Can you work these out from the model? Positions are in its coordinate system, mm. Face numbers are marked on the shaded views. A direction names the side the tool comes from. Round coordinates to 2 decimals unless told otherwise and drop trailing zeros. Order: outer loops, then holes, each group sorted by start corner. A loop starts at its lowest first (then second) coordinate and runs counter-clockwise, first axis right, second up. Notation, with made-up numbers: (89, -18) -> (111, -18) arc R15 cw to (111, 7) -> close; hole circle Ø11 at (20, 15.5). An arc over 180 degrees is marked (long way). Use a Markdown table: item, result. Add a question column.
Q1. We'd pull the mould along X, two halves only. Please class the marked faces 3, 4 and 5: +X half, -X half, draft (parallel to the pull), parting line (faces both ways), or undercut.
Q2. I'm going to push flat-ended pins straight in: pin 1 Ø11.5 at (x, y) = (0, 0) entering from +Z; pin 2 Ø1.5 at (y, z) = (-82.5, -3.5) entering from +X; pin 3 Ø17 at (x, y) = (0, 0) entering from +Z. Where does each tip first touch, or does it pass through?
Q3. For the marked faces 1 and 2, which set-ups out of +Z, -Z, +X, -X, +Y, -Y let a thin tool reach every point of the face, with its end or its side?
Q4. If we section it at A-A on z = 0: List the corners of the cut face in (x, y) for me (3 decimals), plus the area to 3 significant figures.
Q5. I need wall thicknesses on line 1 along Y through (x, z) = (0, -25.5); line 2 along Z through (x, y) = (0, -65.5) (3 decimals); line 3 along Y through (x, z) = (25, 47). Which ranges of each line are inside material? Lowest first, please. Write a range as [from, to].
Q6. If we section it at B-B on y = 71: List the corners of the cut face in (x, z) for me (3 decimals), plus the area to 3 significant figures.
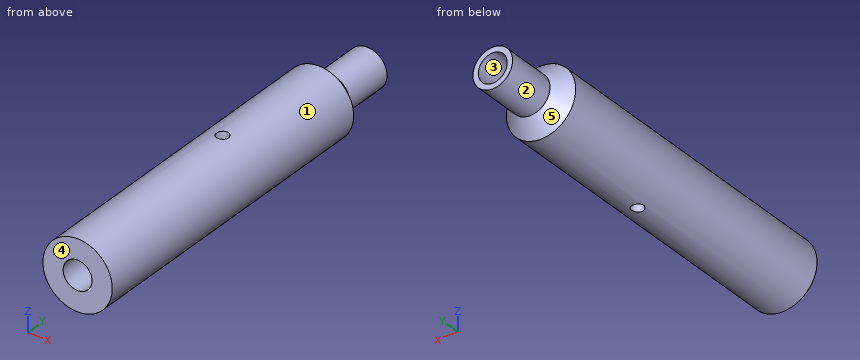
```python
from build123d import *

# Parameters (mm, degrees)
F0_R      = 53.34
F0_R_2    = 22.225
F1_DEPTH  = 304.8
F4_R      = 53.34
F4_R_2    = 30.48
F5_DEPTH  = 101.6
F10_R     = 9.525
F10_R_2   = 3.302
F11_DEPTH = 19.05
F12_DEPTH = 32.3616602869
F13_R     = 9.525
F13_R_2   = 3.302
F14_DEPTH = 19.05
F15_DEPTH = 32.3616602869


with BuildPart() as f1:
    # F0 (on Front) → F1 (new body, symmetric)
    with BuildSketch(Plane.XZ):
        Circle(F0_R)
        Circle(F0_R_2, mode=Mode.SUBTRACT)
    extrude(amount=F1_DEPTH, both=True)

    # F4 (on offset) → F5 (cut)
    with BuildSketch(Plane(origin=(0, 304.8, 0), x_dir=(-1, 0, 0), z_dir=(0, 1, 0))):
        Circle(F4_R)
        Circle(F4_R_2, mode=Mode.SUBTRACT)
    extrude(amount=-F5_DEPTH, mode=Mode.SUBTRACT)

    # F6 (on Right) → F7 (revolve)
    with BuildSketch(Plane.YZ):
        Polygon((203.2, 53.34), (203.2, 30.48), (226.06, 30.48), align=None)
    revolve(axis=Axis((0, 101.6, 0), (0, 1, 0)))

    # F10 (on offset) → F11 (cut)
    with BuildSketch(Plane.XY.offset(53.34)):
        Circle(F10_R)
        Circle(F10_R_2, mode=Mode.SUBTRACT)
        Circle(F10_R_2)
    extrude(amount=-F11_DEPTH, mode=Mode.SUBTRACT)

    # F10 (on offset) → F12 (cut, up to face)
    with BuildSketch(Plane.XY.offset(53.34)):
        Circle(F10_R_2)
    extrude(amount=-F12_DEPTH, mode=Mode.SUBTRACT)

    # F13 (on offset) → F14 (cut)
    with BuildSketch(Plane.XY.offset(-53.34)):
        Circle(F13_R)
        Circle(F13_R_2, mode=Mode.SUBTRACT)
        Circle(F13_R_2)
    extrude(amount=F14_DEPTH, mode=Mode.SUBTRACT)

    # F13 (on offset) → F15 (cut, up to face)
    with BuildSketch(Plane.XY.offset(-53.34)):
        Circle(F13_R_2)
    extrude(amount=F15_DEPTH, mode=Mode.SUBTRACT)

    # F16 (on Right) → F17 (revolve, cut)
    with BuildSketch(Plane.YZ):
        Polygon((6.35, 34.29), (3.302, 34.29), (3.302, 29.21), align=None)
        Polygon((6.35, -34.29), (3.302, -29.21), (3.302, -34.29), align=None)
    revolve(axis=Axis((0, 0, 17.145), (0, 0, 1)), mode=Mode.SUBTRACT)


solid = f1.part
```
Answer below:
| question | item | result |
|---|---|---|
| 1 | face 3 | undercut |
| 1 | face 4 | draft |
| 1 | face 5 | parting line |
| 2 | pin 1 | z = 33.29 |
| 2 | pin 2 | x = 53.27 |
| 2 | pin 3 | z = 34.29 |
| 3 | face 1 | +Y, -Y |
| 3 | face 2 | +Y |
| 4 | outline | (-53.34, -304.8) -> (-22.225, -304.8) -> (-22.225, 304.8) -> (-30.48, 304.8) -> (-30.48, 226.06) -> (-53.34, 203.2) -> close; (22.225, -304.8) -> (53.34, -304.8) -> (53.34, 203.2) -> (30.48, 226.06) -> (30.48, 304.8) -> (22.225, 304.8) -> close |
| 4 | area | 33,800 mm² |
| 5 | line 1 | [-304.8, -3.3], [3.3, 304.8] |
| 5 | line 2 | [-53.34, -22.225], [22.225, 53.34] |
| 5 | line 3 | [-304.8, 203.3] |
| 6 | outline | circle Ø106.68 at (0, 0); hole circle Ø44.45 at (0, 0) |
| 6 | area | 7,390 mm² |
